The model under review builds one solid part; all positions refer to its coordinate system, in mm. Face numbers are marked on the shaded views. A direction names the side the tool comes from. Round coordinates to 2 decimals unless told otherwise and drop trailing zeros. Order: outer loops, then holes, each group sorted by start corner. A loop starts at its lowest first (then second) coordinate and runs counter-clockwise, first axis right, second up.
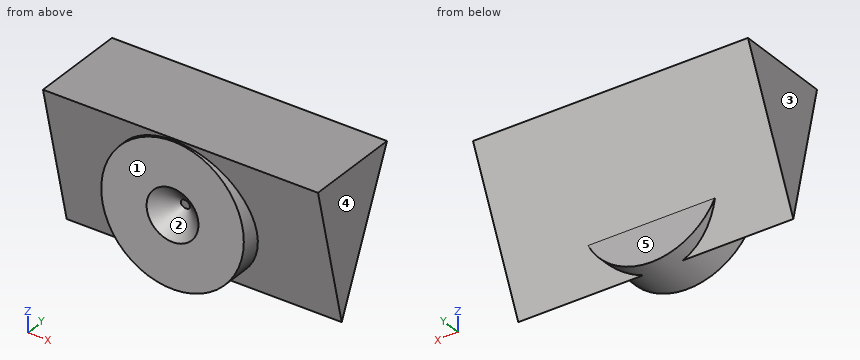
from build123d import *

# Parameters (mm, degrees)
F5_DEPTH = 427.669525


with BuildPart() as f2:
    # F0 (on Top) → F2 (revolve)
    with BuildSketch(Plane.XY):
        Polygon((46.470374, 46.055496), (-0.622407, 0.829846), (39.209366, -33.193126), (109.744787, -33.193126), (109.744787, 46.055496), align=None)
    revolve(axis=Axis((-1.124948, 46.980426, 0), (0, 1, 0)))

    # F4 (on offset) → F5 (join)
    with BuildSketch(Plane.YZ.offset(223.903775)):
        Polygon((120.357007, 113.951385), (-31.448789, 113.951385), (20.660924, -106.508024), align=None)
    extrude(amount=-F5_DEPTH)


solid = f2.part
(1) We need section B-B (y = 3). Give the boundary of the cut face in (x, z).
(2) To check wall thickness, follow L1, parallel to Z at x = -5, y = 39; L2, parallel to Y at x = 70, z = -77.5; L3, parallel to Y at x = 2, z = 80. State the ranges of each line that lie inside material, in increasing order.
(3) Tool access review of the marked faces 4 and 5: name each direction out of +Z, -Z, +X, -X, +Y, -Y from which nothing blocks a thin tool from reaching the whole face with its end or side.
(4) We need section D-D (y = 39). Give the boundary of the cut face in (x, z).
(5) We need section A-A (z = -66.5). Give the boundary of the cut face in (x, y), and give its area (3 significant figures).
(6) We need section C-C (x = -76). Give the boundary of the cut face in (y, z).
(7) The part is to be moulded in two halves that separate along X. For the marked faces 1, 2 and 3, say which applies: pulls with the +X half, pulls with the -X half, needs draft (parallel to the pull), parting line crosses it, or undercut.
(8) Clearance check with flat-ended pins moving along their axes: P1, Ø3, axis at x = 34.5, y = 86.5, coming from the -Z side; P2, Ø18, axis at x = 23.5, z = -77.5, coming from the +Y side; P3, Ø10, axis at x = -93.5, z = -41, coming from the +Y side. State where each tip first meets the part, or that it passes through.
Verdict:
1. outline: (-203.77, -31.79) - (-107.34, -31.79) arc R110.87 ccw to (105.09, -31.79) - (223.9, -31.79) - (223.9, 113.95) - (-203.77, 113.95) - close
2. L1: z = -110.8 to 113.95
2. L2: y = -33.19 to 46.06
2. L3: y = -33.19 to 105
3. face 4: +Z, -Z, +X, +Y, -Y
3. face 5: -Z, +X, -X, +Y
4. outline: (-203.77, -65.95) - (-90.24, -65.95) arc R110.87 ccw to (87.99, -65.95) - (223.9, -65.95) - (223.9, 113.95) - (-203.77, 113.95) - close
5. outline: (-203.77, 11.2) - (-89.84, 11.2) - (-89.84, -33.19) - (87.59, -33.19) - (87.59, 11.2) - (223.9, 11.2) - (223.9, 38.75) - (87.59, 38.75) - (87.59, 46.06) - (-89.84, 46.06) - (-89.84, 38.75) - (-203.77, 38.75) - close
5. area: 21,000 mm2
6. outline: (-33.19, -81.77) - (14.81, -81.77) - (20.66, -106.51) - (31.85, -81.77) - (46.06, -81.77) - (46.06, -50.35) - (120.36, 113.95) - (-31.45, 113.95) - (-23.84, 81.77) - (-33.19, 81.77) - close
7. face 1: needs draft
7. face 2: undercut
7. face 3: pulls with the -X half
8. P1: stops at z = 35.77
8. P2: stops at y = 46.06
8. P3: stops at y = 52.55
